```python
from build123d import *

# Parameters (mm, degrees)
F0_R     = 12.7
F1_DEPTH = 30.1625
F2_W     = 48.26
F2_H     = 22.3266
F3_DEPTH = 22.352
F5_DEPTH = 19.05
F7_DEPTH = 19.05
F8_R     = 6.35
F9_DEPTH = 22.353
F10_R    = 3.302
F11_R    = 7.874
F12_R    = 5.08


with BuildPart() as f1:
    # F0 (on Front) → F1 (new body, symmetric)
    with BuildSketch(Plane.XZ):
        with BuildLine():
            Line((194.2084, 0), (22.352, 0))
            ThreePointArc((22.352, 0), (15.8052507731, -15.8052507731), (0, -22.352))
            Line((0, -22.352), (194.2084, -22.352))
            Line((194.2084, -22.352), (194.2084, 0))
        make_face()
        with BuildLine():
            ThreePointArc((0, -22.352), (15.8052507731, -15.8052507731), (22.352, 0))
            ThreePointArc((22.352, 0), (-15.8052507731, 15.8052507731), (0, -22.352))
        make_face()
        Circle(F0_R, mode=Mode.SUBTRACT)
    extrude(amount=F1_DEPTH, both=True)

    # F2 (on Top) → F3 (cut, symmetric)
    with BuildSketch(Plane.XY):
        with Locations((1.778, 0)):
            Rectangle(F2_W, F2_H)
    extrude(amount=F3_DEPTH, both=True, mode=Mode.SUBTRACT)

    # F4 (on face) → F5 (cut)
    with BuildSketch(Plane.XZ.offset(30.1625)):
        Polygon((85.852, 0), (91.8464, -22.352), (117.2464, -22.352), (117.2464, 0), align=None)
    extrude(amount=-F5_DEPTH, mode=Mode.SUBTRACT)

    # F6 (on face) → F7 (join, through all)
    with BuildSketch(Plane.XZ.offset(30.1625)):
        with BuildLine():
            Line((117.2464, 0), (150.0886, 0))
            Line((150.0886, 0), (150.0886, 34.798))
            Line((150.0886, 34.798), (131.0386, 34.798))
            ThreePointArc((131.0386, 34.798), (127.4644153616, 16.0823576341), (117.2464, 0))
        make_face()
    extrude(amount=-F7_DEPTH)

    # F8 (on face) → F9 (cut, through all)
    with BuildSketch(Plane.XY):
        with Locations((164.3608808517, 7.8105)):
            Circle(F8_R)
    extrude(amount=-F9_DEPTH, mode=Mode.SUBTRACT)

    # F10
    f10_edges = [f1.edges().sort_by_distance(p)[0] for p in [
        (22.352, -20.6629, 0),
        (150.0886, -20.6375, 0),
        (22.352, 20.6629, 0),
    ]]
    fillet(f10_edges, radius=F10_R)

    # F11
    f11_edges = [f1.edges().sort_by_distance(p)[0] for p in [
        (194.2084, 0, 0),
    ]]
    fillet(f11_edges, radius=F11_R)

    # F12
    f12_edges = [f1.edges().sort_by_distance(p)[0] for p in [
        (150.0886, -20.6375, 34.798),
    ]]
    fillet(f12_edges, radius=F12_R)


solid = f1.part
```
Could you check a few things on this model? Use its own coordinates, in mm. A direction names the side the tool comes from. Give positions to 0.01 mm unless a question says otherwise; leave off trailing zeros. Loops run counter-clockwise (first coordinate to the right, second up) from the corner with the lowest first, then second, coordinate; pieces in that order, holes last. Notation, with made-up numbers: (-3, 48.25) - (6, 48.25) arc R26 cw to (6, 68.25) - close; hole circle Ø4 at (15, -23.75). An arc over 180 degrees is marked (long way). Use one line per item in the form item = value.
1. On a 3-axis mill with a long thin cutter (end or side, diameter ignored), from which of +Z, -Z, +X, -X, +Y, -Y can I reach the whole of each face in a straight line? I mean faces 5 (the face through (101, -11.112, -11)), 6 (the face through (139, -11.112, 18)), 7 (the face through (25.908, 0, -11)), 8 (the face through (127.56, -20.77, 16.33)). Say none if no direction works.
Response values:
face_5 = +Z, -Y
face_6 = +Z, +X, -X, +Y
face_7 = +Z, -Z, -X
face_8 = +Z, +Y, -Y
2. I want a section at B-B (y = 21). Please give me the cut outline in (x, z), and give its area (3 significant figures).
Response values:
outline = (0, -22.35) - (194.21, -22.35) - (194.21, -7.87) arc R7.87 ccw to (186.33, 0) - (25.44, 0) arc R3.3 cw to (22.17, 2.88) arc R22.35 ccw (long way) to start; hole circle Ø25.4 at (0, 0)
area = 5,000 mm²
3. I want a section at C-C (z = -3.5). Please give me the cut outline in (x, y).
Response values:
outline = (-22.08, -30.16) - (-12.21, -30.16) - (-12.21, -11.16) - (-22.08, -11.16) - close; (-22.08, 11.16) - (-12.21, 11.16) - (-12.21, 30.16) - (-22.08, 30.16) - close; (12.21, -30.16) - (86.79, -30.16) - (86.79, -11.11) - (117.25, -11.11) - (117.25, -30.16) - (192.88, -30.16) - (192.88, 30.16) - (12.21, 30.16) - (12.21, 11.16) - (25.91, 11.16) - (25.91, -11.16) - (12.21, -11.16) - close; hole circle Ø12.7 at (164.36, 7.81)
4. Thinking about a two-plate mould opening in Z: for faces 1 (the face through (-2.75, 20.8, -12.4)), 2 (the face through (12, -11.163, -5)), 3 (the face through (-16.31, 20.53, 15.284)), 4 (the face through (107, 6, 0)), which applies, released by +Z, released by -Z, zero draft, split by the parting line, or undercut?
Response values:
face_1 = undercut
face_2 = zero draft
face_3 = split by the parting line
face_4 = released by +Z
5. I need wall thicknesses on probe 1 along Y at (x, z) = (21, 4); probe 2 along X at (y, z) = (12.5, -7.5); probe 3 along Z at (x, y) = (177, 21). Which ranges of each line are inside material? Lowest first, please.
Response values:
probe_1 = -30.16 to -11.16, 11.16 to 30.16
probe_2 = -21.06 to -10.25, 10.25 to 160.08, 168.64 to 194.2
probe_3 = -22.35 to 0
6. I want a section at A-A (y = -16.5). Please give me the cut outline in (x, z).
Response values:
outline = (0, -22.35) - (91.85, -22.35) - (85.85, 0) - (25.44, 0) arc R3.3 cw to (22.17, 2.88) arc R22.35 ccw (long way) to start; (117.25, -22.35) - (194.21, -22.35) - (194.21, -7.87) arc R7.87 ccw to (186.33, 0) - (153.39, 0) arc R3.3 cw to (150.09, 3.3) - (150.09, 29.72) arc R5.08 ccw to (145.01, 34.8) - (131.04, 34.8) arc R50.8 cw to (117.25, 0) - close; hole circle Ø25.4 at (0, 0)
7. I'm going to push flat-ended pins straight in: pin 1 Ø4 at (x, y) = (86, 14.5) entering from +Z; pin 2 Ø20.5 at (x, y) = (164.36, 7.81) entering from -Z; pin 3 Ø9.5 at (y, z) = (-20.5, -12) entering from -X; pin 4 Ø11 at (y, z) = (-3, -14.5) entering from -X. Where does each tip first touch, or does it pass through?
Response values:
pin_1 = 0
pin_2 = -22.35
pin_3 = -21.14
pin_4 = 25.91
8. I want a section at D-D (z = -16). Please give me the cut outline in (x, y), and give its area (3 significant figures).
Response values:
outline = (-15.61, -30.16) - (90.14, -30.16) - (90.14, -11.11) - (117.25, -11.11) - (117.25, -30.16) - (194.21, -30.16) - (194.21, 30.16) - (-15.61, 30.16) - (-15.61, 11.16) - (25.91, 11.16) - (25.91, -11.16) - (-15.61, -11.16) - close; hole circle Ø12.7 at (164.36, 7.81)
area = 11,100 mm²
